Source: CAD feature listing. Evaluate the final solid. Frame: model axes, mm. A direction names the side the tool comes from. Give positions to 0.01 mm unless a question says otherwise; leave off trailing zeros. Loops run counter-clockwise (first coordinate to the right, second up) from the corner with the lowest first, then second, coordinate; pieces in that order, holes last. Notation, with made-up numbers: (5, -6) -> (19, -6) arc R21 cw to (19, 27) -> close; hole circle Ø2 at (-25.5, 0.5). An arc over 180 degrees is marked (long way). Put each result on its own line as item: value.
```python
from build123d import *

# Parameters (mm, degrees)
F0_R     = 5.4
F1_DEPTH = 3.5
F2_R     = 6
F2_R_2   = 5.4
F3_DEPTH = 0.5
F4_R     = 4.75
F5_DEPTH = 3
F7_R     = 1.75
F8_DEPTH = 0.5
F9_R     = 0.75
F6_R     = 0.7


with BuildPart() as f1:
    # F0 (on Front) → F1 (new body)
    with BuildSketch(Plane.XZ):
        Circle(F0_R)
    extrude(amount=F1_DEPTH)

    # F2 (on face) → F3 (join)
    with BuildSketch(Plane(origin=(0, 0, 0), x_dir=(-1, 0, 0), z_dir=(0, 1, 0))):
        Circle(F2_R)
        Circle(F2_R_2, mode=Mode.SUBTRACT)
        Circle(F2_R_2)
    extrude(amount=F3_DEPTH)

    # F4 (on face) → F5 (cut)
    with BuildSketch(Plane(origin=(0, 0.5, 0), x_dir=(-1, 0, 0), z_dir=(0, 1, 0))):
        Circle(F4_R)
    extrude(amount=-F5_DEPTH, mode=Mode.SUBTRACT)

    # F7 (on face) → F8 (join)
    with BuildSketch(Plane(origin=(0, -2.5, 0), x_dir=(-1, 0, 0), z_dir=(0, 1, 0))):
        Circle(F7_R)
    extrude(amount=F8_DEPTH)

    # F9 (on face) → F10 section 0
    with BuildSketch(Plane(origin=(0, -2, 0), x_dir=(-1, 0, 0), z_dir=(0, 1, 0))):
        Circle(F9_R)
    # F6 (on face) → F10 section 1
    with BuildSketch(Plane.XZ.offset(3.5)):
        Circle(F6_R)
    loft(mode=Mode.SUBTRACT)


solid = f1.part
```
(1) Section C-C on y = -2.15. Return loops of the section in (x, z) (3 decimals), then the cut area to 3 significant figures.
Calculated:
outline: circle Ø10.8 at (0, 0); circle Ø3.5 at (0, 0); hole circle Ø9.5 at (0, 0); hole circle Ø1.49 at (0, 0)
area: 28.6 mm²
(2) Section B-B on y = -1.1. Return loops of the section in (x, z), then the cut area to 3 significant figures.
Calculated:
outline: circle Ø10.8 at (0, 0); hole circle Ø9.5 at (0, 0)
area: 20.7 mm²
(3) Line query: probe 1 along Z at (x, y) = (0, -0.3); probe 2 along Y at (x, z) = (-1.5, -1.5); probe 3 along Y at (x, z) = (1.25, 5.5). Output: solid intervals per line, ascending. Write a range as from..to.
Calculated:
probe 1: z = -5.4..-4.75, 4.75..5.4
probe 2: y = -3.5..-2.5
probe 3: y = 0..0.5
(4) Reachability of faces 5 (the cylindrical face through (-2.192, -0.979, -4.214)), 6 (the flat face through (0, -3.5, -1)) from +Z, -Z, +X, -X, +Y, -Y: full face, straight path, thin tool, end or side. Return the list, or none.
Calculated:
face 5: +Y
face 6: +Z, -Z, +X, -X, -Y
(5) First-contact query: P1, Ø1, axis at y = -1, z = 1, coming from the +X side; P2, Ø3, axis at x = 0, z = 2, coming from the +Y side. Flat tips, straight axial feed; report the tip coordinate or a pass-through.
Calculated:
P1: stops at x = 5.38
P2: stops at y = -2
(6) Draft query along X for faces 1 (the flat face through (-4, 0.5, -3)), 2 (the flat face through (-2, -2.5, 0)), 3 (the conical face through (-0.69, -2.76, 0.22)), 4 (the cylindrical face through (-1.17, -1.73, -5.27)). Return one class per face: released by +X, released by -X, zero draft, split by the parting line, or undercut.
Calculated:
face 1: zero draft
face 2: undercut
face 3: undercut
face 4: split by the parting line
(7) Section D-D on z = -4.5. Return loops of the section in (x, y), then the cut area to 3 significant figures.
Calculated:
outline: (-3.97, 0) -> (-2.98, 0) -> (-2.98, -3.5) -> (2.98, -3.5) -> (2.98, 0) -> (3.97, 0) -> (3.97, 0.5) -> (1.52, 0.5) -> (1.52, -2.5) -> (-1.52, -2.5) -> (-1.52, 0.5) -> (-3.97, 0.5) -> close
area: 15.7 mm²
(8) Section A-A on x = 0. Return loops of the section in (y, z), then the cut area to 3 significant figures.
Calculated:
outline: (-3.5, -5.4) -> (0, -5.4) -> (0, -6) -> (0.5, -6) -> (0.5, -4.75) -> (-2.5, -4.75) -> (-2.5, -1.75) -> (-2, -1.75) -> (-2, -0.75) -> (-3.5, -0.7) -> close; (-3.5, 0.7) -> (-2, 0.75) -> (-2, 1.75) -> (-2.5, 1.75) -> (-2.5, 4.75) -> (0.5, 4.75) -> (0.5, 6) -> (0, 6) -> (0, 5.4) -> (-3.5, 5.4) -> close
area: 14.9 mm²
